```python
from build123d import *

# Parameters (mm, degrees)
F0_W     = 71.666194126
F0_H     = 28.7182237953
F1_DEPTH = 5
F2_R     = 5.08
F3_R     = 5.08
F4_R     = 5.08
F5_R     = 5.08
F6_T     = -1
F7_R     = 1


with BuildPart() as f1:
    # F0 (on Top) → F1 (new body)
    with BuildSketch(Plane.XY):
        with Locations((-18.4986749664, 23.9965328947)):
            Rectangle(F0_W, F0_H)
    extrude(amount=F1_DEPTH)

    # F2
    f2_edges = [f1.edges().sort_by_distance(p)[0] for p in [
        (-54.331772, 38.355645, 2.5),
    ]]
    fillet(f2_edges, radius=F2_R)

    # F3
    f3_edges = [f1.edges().sort_by_distance(p)[0] for p in [
        (-54.331772, 9.637421, 2.5),
    ]]
    fillet(f3_edges, radius=F3_R)

    # F4
    f4_edges = [f1.edges().sort_by_distance(p)[0] for p in [
        (17.334422, 9.637421, 2.5),
    ]]
    fillet(f4_edges, radius=F4_R)

    # F5
    f5_edges = [f1.edges().sort_by_distance(p)[0] for p in [
        (17.334422, 38.355645, 2.5),
    ]]
    fillet(f5_edges, radius=F5_R)

    # F6
    f6_openings = [f1.faces().sort_by_distance(p)[0] for p in [
        (-18.498675, 23.996533, 5),
    ]]
    offset(amount=F6_T, openings=f6_openings)

    # F7
    f7_edges = [f1.edges().sort_by_distance(p)[0] for p in [
        (-52.136768, 11.832425, 1),
        (-18.498675, 10.637421, 1),
        (15.139418, 11.832425, 1),
        (16.334422, 23.996533, 1),
        (15.139418, 36.16064, 1),
        (-18.498675, 37.355645, 1),
        (-52.136768, 36.16064, 1),
        (-53.331772, 23.996533, 1),
    ]]
    fillet(f7_edges, radius=F7_R)


solid = f1.part
```
CAD build for the part. Positions are in the model's coordinates, mm. A direction names the side the tool comes from. Coordinates: 2 decimals unless noted, no trailing zeros. Order: outer loops, then holes, each group sorted by start corner. A loop starts at its lowest first (then second) coordinate and runs counter-clockwise, first axis right, second up.
(1) Saw through at C-C, the plane y = 21.25. Write the cut outline in (x, z).
Solution:
outline: (-54.33, 0) - (17.33, 0) - (17.33, 5) - (16.33, 5) - (16.33, 2) arc R1 cw to (15.33, 1) - (-52.33, 1) arc R1 cw to (-53.33, 2) - (-53.33, 5) - (-54.33, 5) - close
(2) Mould opens along X. For faces 3 (the face through (-52.883, 11.165, 2.535)), 4 (the face through (15.108, 11.801, 3.521)), 5 (the face through (15.2, 36.1, 3.5)), 6 (the face through (17.334, 24, 2)) say: released by +X, released by -X, zero draft, split by the parting line, or undercut.
Solution:
face 3: released by -X
face 4: undercut
face 5: undercut
face 6: released by +X
(3) Saw through at B-B, the plane x = -40.5. Write the cut outline in (y, z).
Solution:
outline: (9.64, 0) - (38.36, 0) - (38.36, 5) - (37.36, 5) - (37.36, 2) arc R1 cw to (36.36, 1) - (11.64, 1) arc R1 cw to (10.64, 2) - (10.64, 5) - (9.64, 5) - close
(4) Drill centre lines: L1, parallel to Y at x = 3.5, z = 3.7; L2, parallel to X at y = 26.75, z = 1.95; L3, parallel to Z at x = -22, y = 15. Where is each one in solid material? Low to high.
Solution:
L1: y = 9.64 to 10.64, 37.36 to 38.36
L2: x = -54.33 to -53.33, 16.33 to 17.33
L3: z = 0 to 1
(5) Which spindle directions (+Z, -Z, +X, -X, +Y, -Y) get a long thin tool onto all of the face, cutting with end or side? Do faces 1 (the face through (-52.168, 11.864, 3.521)), 2 (the face through (15.81, 11.09, 2.54)). Say none if no direction does.
Solution:
face 1: +Z
face 2: +Z, -Z, +X, -Y
(6) Saw through at A-A, the plane z = 3.1. Write the cut outline in (x, y).
Solution:
outline: (-54.33, 14.72) arc R5.08 ccw to (-49.25, 9.64) - (12.25, 9.64) arc R5.08 ccw to (17.33, 14.72) - (17.33, 33.28) arc R5.08 ccw to (12.25, 38.36) - (-49.25, 38.36) arc R5.08 ccw to (-54.33, 33.28) - close; hole (-53.33, 14.72) arc R4.08 ccw to (-49.25, 10.64) - (12.25, 10.64) arc R4.08 ccw to (16.33, 14.72) - (16.33, 33.28) arc R4.08 ccw to (12.25, 37.36) - (-49.25, 37.36) arc R4.08 ccw to (-53.33, 33.28) - close
(7) Pin check, flat tip, straight feed: pin 1 Ø12.5 at (x, y) = (-31, 23) entering from +Z. Stop position of the tip, or through.
Solution:
pin 1: stops at z = 1
